Verification items for the finished model (mm, model axes). A direction names the side the tool comes from. Give positions to 0.01 mm unless a question says otherwise; leave off trailing zeros. Loops run counter-clockwise (first coordinate to the right, second up) from the corner with the lowest first, then second, coordinate; pieces in that order, holes last. Notation, with made-up numbers: (41, 61.5) - (98, 61.5) arc R15 ccw to (98, 79.5) - close; hole circle Ø7 at (46.25, 28.25). An arc over 180 degrees is marked (long way). One line per item, written item: value. Start each with the question number.
1. Sectioned sample at C-C (x = 212). Record the cut outline in (y, z), plus the area to 3 significant figures.
2. Scan lines: L1, parallel to X at y = -7.5, z = 9; L2, parallel to X at y = -10, z = 16; L3, parallel to Y at x = -9, z = 2. Record each from-to range of solid material in increasing order. Write a range as [from, to].
3. Gauge pin test, flat ends, axial feed: pin 1 (1.5 mm diameter, centred on x = 304, z = 9, fed in from -Y); pin 2 (12 mm diameter, centred on x = 141, z = 13, fed in from -Y); pin 3 (10 mm diameter, centred on y = -2, z = -15, fed in from +X); pin 4 (1.5 mm diameter, centred on x = 277.5, z = 12.5, fed in from +Y). Record the tip position at first contact, or that the pin passes through.
4. Sectioned sample at A-A (z = 0). Record the cut outline in (x, y).
5. Access from +Z, -Z, +X, -X, +Y, -Y to the whole of each face (thin tool, end or side, straight path). Record for faces 1 (the flat face through (-27, 0, 7.5)), 2 (the flat face through (-27, -7.5, 0)), 3 (the flat face through (12, -4, 12.4)), 4 (the flat face through (-27, 7.5, 0)).
from build123d import *

# Parameters (mm, degrees)
SKETCH2_W           = 15
SKETCH2_H           = 15
BOSS_EXTRUDE1_DEPTH = 35


with BuildPart() as part:
    # Sketch1 → Revolve1 (revolve)
    with BuildSketch(Plane.XY, mode=Mode.PRIVATE) as revolve1_sk:
        with BuildLine():
            Line((0, 19), (12, 19))
            Line((12, 19), (12, 12.5))
            Line((12, 12.5), (269, 12.5))
            Line((269, 12.5), (269, 10))
            Line((269, 10), (352, 10))
            ThreePointArc((352, 10), (359.071067812, 7.071067812), (362, 0))
            Line((362, 0), (-10, 0))
            Line((-10, 0), (-10, 12.5))
            ThreePointArc((-10, 12.5), (-4.143637104, 14.432518621), (0, 19))
        make_face()
    revolve(revolve1_sk.sketch.rotate(Axis((-14.332813636, 0, 0), (1, 0, 0)), 180), axis=Axis((-14.332813636, 0, 0), (1, 0, 0)))

    # Sketch2 → Boss-Extrude1 (add)
    with BuildSketch(Plane.ZY.offset(10)):
        Rectangle(SKETCH2_W, SKETCH2_H)
    extrude(amount=BOSS_EXTRUDE1_DEPTH)


solid = part.part
Results are:
1. outline: circle Ø25 at (0, 0)
1. area: 491 mm^2
2. L1: x = [-10, 269]
2. L2: x = [-0.07, 12]
2. L3: y = [-12.44, 12.44]
3. pin 1: stops at y = -5.65
3. pin 2: stops at y = -10.36
3. pin 3: stops at x = 269
3. pin 4: passes through
4. outline: (-45, -7.5) - (-10, -7.5) - (-10, -12.5) arc R12.1 cw to (0, -19) - (12, -19) - (12, -12.5) - (269, -12.5) - (269, -10) - (352, -10) arc R10 ccw to (352, 10) - (269, 10) - (269, 12.5) - (12, 12.5) - (12, 19) - (0, 19) arc R12.1 cw to (-10, 12.5) - (-10, 7.5) - (-45, 7.5) - close
5. face 1: +Z, -X, +Y, -Y
5. face 2: +Z, -Z, -X, -Y
5. face 3: +X
5. face 4: +Z, -Z, -X, +Y
